Here's how the part is built. I have some questions about the finished solid (model axes, mm). Face numbers are marked on the shaded views. A direction names the side the tool comes from. Coordinates: 2 decimals unless noted, no trailing zeros. Write each loop counter-clockwise with the first axis right and the second up, starting at its lowest first coordinate (ties: lowest second). Pieces come first, ordered by that corner, then holes.
```python
from build123d import *

# Parameters (mm, degrees)
F0_R      = 12.7
F1_DEPTH  = 20.32
F3_R      = 9.525
F4_DEPTH  = 3.175
F4_TAPER  = -45
F6_R      = 6.477
F7_DEPTH  = 23.496
F8_W      = 31.75
F8_H      = 25.908
F9_DEPTH  = 4.572
F11_R     = 6.477
F12_DEPTH = 28.068
F14_R     = 7.8994
F15_DEPTH = 25.909


with BuildPart() as f1:
    # F0 (on Top) → F1 (new body)
    with BuildSketch(Plane.XY):
        Circle(F0_R)
    extrude(amount=F1_DEPTH)

    # F3 (on offset) → F4 (join)
    with BuildSketch(Plane.XY.offset(20.32)):
        Circle(F3_R)
    extrude(amount=F4_DEPTH, taper=F4_TAPER)

    # F6 (on offset) → F7 (cut, through all)
    with BuildSketch(Plane.XY.offset(23.495)):
        Circle(F6_R)
    extrude(amount=-F7_DEPTH, mode=Mode.SUBTRACT)

    # F8 (on offset) → F9 (join)
    with BuildSketch(Plane.XY.offset(23.495)):
        Rectangle(F8_W, F8_H)
    extrude(amount=F9_DEPTH)

    # F11 (on offset) → F12 (cut, through all)
    with BuildSketch(Plane.XY.offset(28.067)):
        Circle(F11_R)
    extrude(amount=-F12_DEPTH, mode=Mode.SUBTRACT)

    # F14 (on offset) → F15 (cut, through all)
    with BuildSketch(Plane.XZ.offset(12.954)):
        with Locations((0, 32.1564)):
            Circle(F14_R)
    extrude(amount=-F15_DEPTH, mode=Mode.SUBTRACT)


solid = f1.part
```
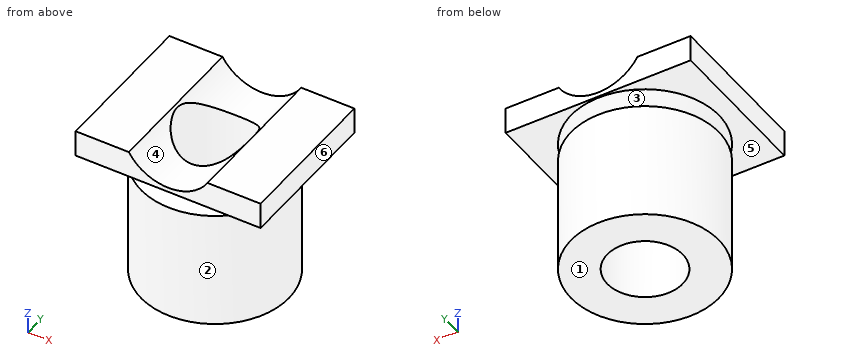
1) Imagine slicing it at C-C on z = 9.5. Please give me the cut outline in (x, y), then the cut area to 3 significant figures.
Values follow:
outline: circle Ø25.4 at (0, 0); hole circle Ø12.95 at (0, 0)
area: 375 mm2
2) I need wall thicknesses on probe 1 along Y at (x, z) = (0, 15.75); probe 2 along Y at (x, z) = (5, 2); probe 3 along Z at (x, y) = (0, -11.5) (3 decimals). Which ranges of each line are inside material? Lowest first, please.
Values follow:
probe 1: y = -12.7 to -6.48, 6.48 to 12.7
probe 2: y = -11.67 to -4.12, 4.12 to 11.67
probe 3: z = 0 to 20.32, 22.295 to 24.257
3) Imagine slicing it at B-B on x = 0. Please give me the cut outline in (y, z) (3 decimals).
Values follow:
outline: (-12.954, 23.495) - (-12.7, 23.495) - (-9.525, 20.32) - (-12.7, 20.32) - (-12.7, 0) - (-6.477, 0) - (-6.477, 24.257) - (-12.954, 24.257) - close; (6.477, 0) - (12.7, 0) - (12.7, 20.32) - (9.525, 20.32) - (12.7, 23.495) - (12.954, 23.495) - (12.954, 24.257) - (6.477, 24.257) - close
4) Will these pins go through, and if not, where does the flat tip stop? pin 1 (15 mm diameter, centred on x = 0, y = 0, fed in from +Z); pin 2 (6 mm diameter, centred on x = -5, z = 13.5, fed in from -Y); pin 3 (1.5 mm diameter, centred on x = -4, z = 3.5, fed in from +Y); pin 4 (5 mm diameter, centred on y = -6, z = 13, fed in from +X).
Values follow:
pin 1: stops at z = 28.07
pin 2: stops at y = -12.54
pin 3: stops at y = 12.28
pin 4: stops at x = 12.21
5) We'd pull the mould along Z, two halves only. Please class the marked faces 3, 4, 5 and 6: pulls with the +Z half, pulls with the -Z half, needs draft (parallel to the pull), parting line crosses it, or undercut.
Values follow:
face 3: undercut
face 4: pulls with the +Z half
face 5: pulls with the -Z half
face 6: needs draft
6) Imagine slicing it at A-A on z = 26.25. Please give me the cut outline in (x, y) (3 decimals), then the cut area to 3 significant figures.
Values follow:
outline: (-15.875, -12.954) - (-5.245, -12.954) - (-5.245, -3.8) arc R6.477 cw to (-5.245, 3.8) - (-5.245, 12.954) - (-15.875, 12.954) - close; (5.245, -12.954) - (15.875, -12.954) - (15.875, 12.954) - (5.245, 12.954) - (5.245, 3.8) arc R6.477 cw to (5.245, -3.8) - close
area: 538 mm2
7) Imagine slicing it at D-D on z = 21.5. Please give me the cut outline in (x, y) (3 decimals).
Values follow:
outline: circle Ø21.41 at (0, 0); hole circle Ø12.954 at (0, 0)
8) On a 3-axis mill with a long thin cutter (end or side, diameter ignored), from which of +Z, -Z, +X, -X, +Y, -Y can I reach the whole of each face in a straight line? I mean the marked faces 1 and 2. Say none if no direction works.
Values follow:
face 1: -Z, +X, -X, +Y, -Y
face 2: -Z
